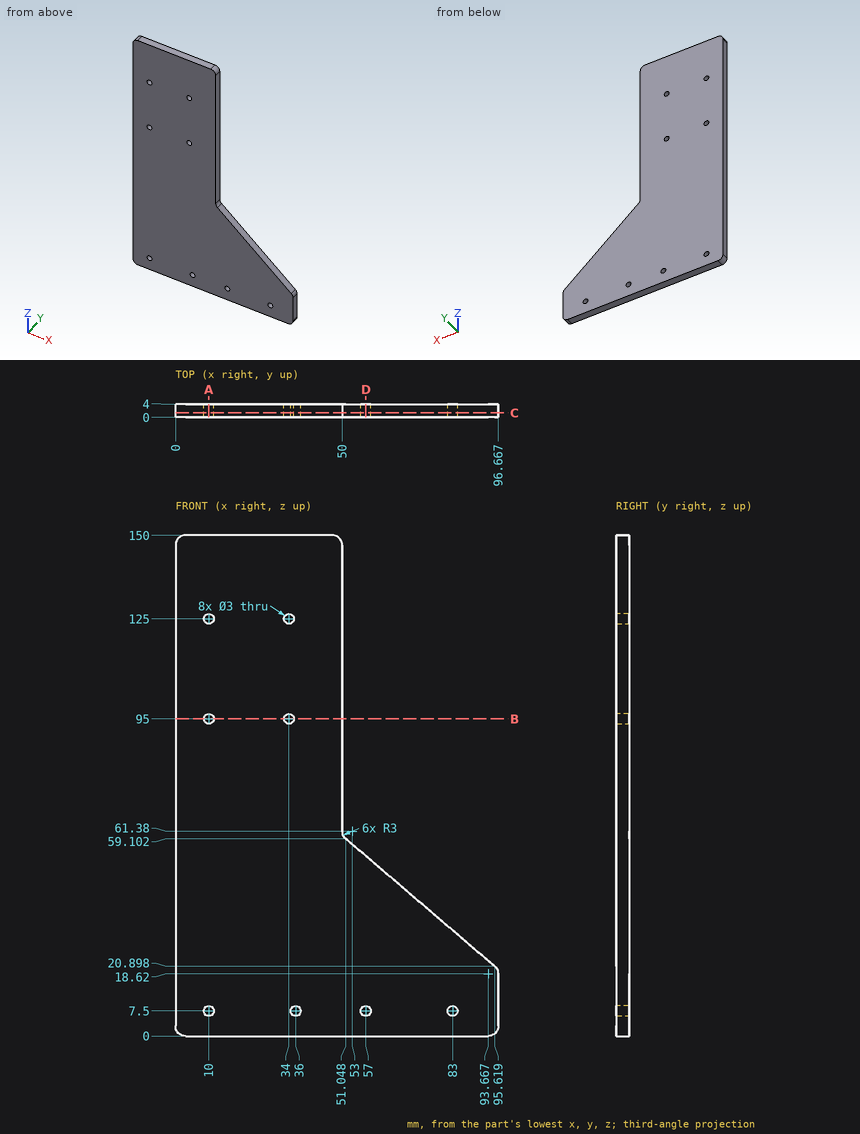
Print and shaded views of the part. All mm, measured from the part's lowest x, y and z. Round coordinates to 2 decimals unless told otherwise and drop trailing zeros. Write each loop counter-clockwise with the first axis right and the second up, starting at its lowest first coordinate (ties: lowest second). Pieces come first, ordered by that corner, then holes. Notation, with made-up numbers: M 14.5,65.5 L 54.5,65.5 A32 cw 54.5,101.5 Z; hole C 27.25,-30.75 d8. An arc over 180 degrees is marked long. One line per question, with ' | ' between items.
(1) Saw through at D-D on x = 57. Write the cut outline in (y, z).
Answer key:
outline: M 0,0 L 4,0 L 4,6 L 0,6 Z; M 0,9 L 4,9 L 4,54 L 0,54 Z
(2) Pin check, flat tips, straight feed: pin 1 (1.5 mm diameter, centred on y = 3.5, z = 99.5, fed in from -X); pin 2 (2.5 mm diameter, centred on x = 83, z = 7.5, fed in from +Y). Stop position of each tip, or through.
Answer key:
pin 1: stops at x = 0 | pin 2: passes through
(3) Saw through at A-A on x = 10. Write the cut outline in (y, z).
Answer key:
outline: M 0,0 L 4,0 L 4,6 L 0,6 Z; M 0,9 L 4,9 L 4,93.5 L 0,93.5 Z; M 0,96.5 L 4,96.5 L 4,123.5 L 0,123.5 Z; M 0,126.5 L 4,126.5 L 4,150 L 0,150 Z
(4) Saw through at C-C on y = 1.35. Count the separate pieces of the cut face and the enclosed holes in it, then the cut area to 3 significant figures.
Answer key:
separate pieces: 1 | enclosed holes: 8 | area: 9,300 mm^2
(5) Saw through at B-B on z = 95. Write the cut outline in (x, y).
Answer key:
outline: M 0,0 L 8.5,0 L 8.5,4 L 0,4 Z; M 11.5,0 L 32.5,0 L 32.5,4 L 11.5,4 Z; M 35.5,0 L 50,0 L 50,4 L 35.5,4 Z
(6) Probe line 1 along X through (y, z) = (0.9, 95); line 2 along X through (y, z) = (1, 7.5); line 3 along X through (y, z) = (2.3, 99.5). List the from-to ranges inside material, lowest first.
Answer key:
line 1: x = 0 to 8.5, 11.5 to 32.5, 35.5 to 50 | line 2: x = 0 to 8.5, 11.5 to 34.5, 37.5 to 55.5, 58.5 to 81.5, 84.5 to 96.67 | line 3: x = 0 to 50
